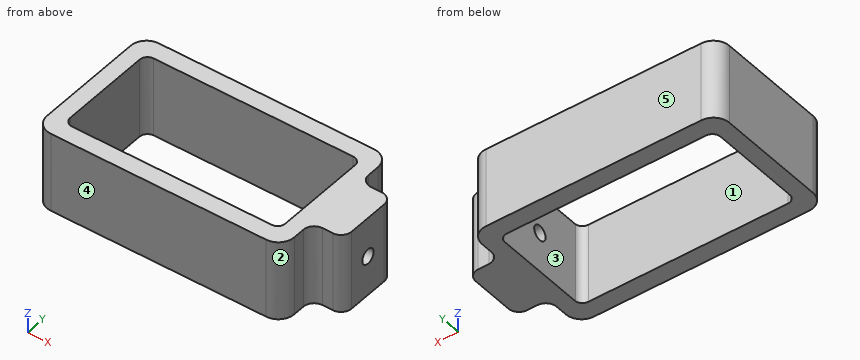
Autodesk Inventor part; units mm, degrees
ref_plane "YZ Plane" through (0, 0, 0) normal (1, 0, 0) x (0, 1, 0)
ref_plane "XZ Plane" through (0, 0, 0) normal (0, 1, 0) x (-1, 0, 0)
ref_plane "Arbeitsebene1" through (0, 0, -15) normal (0, 0, 1) x (1, 0, 0)
sketch "Skizze1" plane through (0, 0, -15) normal (0, 0, 1) x (1, 0, 0)
  line L0 (29.6698, 8.5) -> (29.6698, -8.5)
  arc A0 (29.6698, 8.5) -> (28.1698, 10) centre (28.1698, 8.5) ccw
  line L1 (11.1698, 10) -> (28.1698, 10)
  arc A1 (11.1698, 10) -> (9.6698, 8.5) centre (11.1698, 8.5) ccw
  line L2 (9.6698, -8.5) -> (9.6698, 8.5)
  arc A2 (9.6698, -8.5) -> (11.1698, -10) centre (11.1698, -8.5) ccw
  line L3 (28.1698, -10) -> (11.1698, -10)
  arc A3 (28.1698, -10) -> (29.6698, -8.5) centre (28.1698, -8.5) ccw
  circle A4 centre (27.6698, 8) radius 0.7835
  circle A5 centre (27.6698, -8) radius 0.7835
  circle A6 centre (11.6698, 8) radius 0.7835
  circle A7 centre (11.6698, -8) radius 0.7835
  circle A8 centre (19.6698, 0) radius 7.5
  line L4 (4.2698, 10) -> (4.2698, 8.9)
  line L5 (-5.8302, 10) -> (4.2698, 10)
  line L6 (-5.8302, 8.5) -> (-5.8302, 10)
  arc A9 (-9.3302, 5) -> (-5.8302, 8.5) centre (-9.3302, 8.5) ccw
  line L7 (-10.8302, 5) -> (-9.3302, 5)
  line L8 (-10.8302, -5) -> (-10.8302, 5)
  line L9 (-9.3302, -5) -> (-10.8302, -5)
  arc A10 (-5.8302, -8.5) -> (-9.3302, -5) centre (-9.3302, -8.5) ccw
  line L10 (-5.8302, -10) -> (-5.8302, -8.5)
  line L11 (4.2698, -10) -> (-5.8302, -10)
  line L12 (4.2698, -8.9) -> (4.2698, -10)
  arc A11 (7.6698, -5.5) -> (4.2698, -8.9) centre (7.6698, -8.9) ccw
  line L13 (11.1698, -5.5) -> (7.6698, -5.5)
  line L14 (11.1698, -5) -> (11.1698, -5.5)
  line L15 (11.1698, -5) -> (7.3698, -5)
  line L16 (7.3698, -5) -> (7.3698, 5)
  line L17 (7.3698, 5) -> (11.1698, 5)
  line L18 (11.1698, 5.5) -> (11.1698, 5)
  line L19 (7.6698, 5.5) -> (11.1698, 5.5)
  arc A12 (4.2698, 8.9) -> (7.6698, 5.5) centre (7.6698, 8.9) ccw
  circle A13 centre (-0.8302, 0) radius 2
  line L20 (9.1698, 8.5) -> (9.1698, -8.5)
  arc A14 (9.1698, 8.5) -> (7.6698, 10) centre (7.6698, 8.5) ccw
  line L21 (-9.3302, 10) -> (7.6698, 10)
  arc A15 (-9.3302, 10) -> (-10.8302, 8.5) centre (-9.3302, 8.5) ccw
  line L22 (-10.8302, -8.5) -> (-10.8302, 8.5)
  arc A16 (-10.8302, -8.5) -> (-9.3302, -10) centre (-9.3302, -8.5) ccw
  line L23 (7.6698, -10) -> (-9.3302, -10)
  arc A17 (7.6698, -10) -> (9.1698, -8.5) centre (7.6698, -8.5) ccw
  circle A18 centre (7.1698, 8) radius 0.7835
  circle A19 centre (7.1698, -8) radius 0.7835
  circle A20 centre (-8.8302, 8) radius 0.7835
  circle A21 centre (-8.8302, -8) radius 0.7835
  circle A22 centre (-0.8302, 0) radius 7.5
  line L24 (-9.3302, -5.5) -> (-12.8302, -5.5)
  line L25 (-9.3302, -5) -> (-9.3302, -5.5)
  line L26 (-9.3302, -5) -> (-13.1302, -5)
  line L27 (-13.1302, 5) -> (-9.3302, 5)
  line L28 (-9.3302, 5.5) -> (-9.3302, 5)
  line L29 (-12.8302, 5.5) -> (-9.3302, 5.5)
  line L30 (11.1698, 10) -> (7.6698, 10)
  line L31 (11.1698, -10) -> (7.6698, -10)
  line L32 (-10.858, 10.25) -> (29.642, 10.25)
  line L33 (29.642, 10.25) -> (29.642, -10.25)
  line L34 (29.642, -10.25) -> (-10.858, -10.25)
  line L35 (-10.858, -10.25) -> (-10.858, 10.25)
  line L36 (-10.858, 10.25) -> (29.642, -10.25) construction
  line L37 (29.642, 10.25) -> (-10.858, -10.25) construction
  line L38 (32.642, -10.25) -> (32.642, 10.25)
  line L39 (29.642, 13.25) -> (-10.858, 13.25)
  line L40 (-13.858, 10.25) -> (-13.858, -10.25)
  line L41 (-10.858, -13.25) -> (29.642, -13.25)
  arc A23 (32.642, 10.25) -> (29.642, 13.25) centre (29.642, 10.25) ccw
  arc A24 (29.642, -13.25) -> (32.642, -10.25) centre (29.642, -10.25) ccw
  arc A25 (-13.858, -10.25) -> (-10.858, -13.25) centre (-10.858, -10.25) ccw
  arc A26 (-10.858, 13.25) -> (-13.858, 10.25) centre (-10.858, 10.25) ccw
  line L42 (38.642, 6) -> (32.642, 6)
  line L43 (32.642, 6) -> (32.642, -6)
  line L44 (32.642, -6) -> (38.642, -6)
  line L45 (38.642, -6) -> (38.642, 6)
  line L46 (38.642, 6) -> (32.642, -6) construction
  line L47 (32.642, 6) -> (38.642, -6) construction
  point P0 (0, 0)
  point P1 (9.392, 0)
  point P2 (35.642, 0)
  point P3 (32.642, 0)
  point P4 (29.642, -8.7873)
  point P5 (29.642, 8.7873)
  dimension "d1" = 20.5
  dimension "d2" = 3
  dimension "d3" = 3
  dimension "d6" = 6
  dimension "d7" = 12
extrude "Extrusion1" add sketch "Skizze1" along normal blind 15 contours L0 A3 L33 A0 | A0 L1 L30 L21 L5 A15 L22 L29 L35 L32 L33 | L33 L34 L35 L24 L22 A16 L23 L11 L31 L3 A3 | L29 L22 L27 L35 | L35 L26 L22 L24 | L27 L8 L26 L35 | A24 L41 A25 L40 A26 L39 A23 L38 | L38 L42 L45 L44
fillet "Rundung1" radius 2 4 edges at (32.642, 6, -7.5) (38.642, 6, -7.5) (38.642, -6, -7.5) (32.642, -6, -7.5)
sketch "Skizze2" plane through (38.642, -4, -15) normal (1, 0, 0) x (0, 0, -1)
  line L0 (0, 0) -> (-15, 0)
  line L1 (0, 0) -> (0, 8)
  line L2 (-15, 8) -> (0, 8)
  line L3 (-15, 0) -> (-15, 8)
  circle A0 centre (-7.5, 4) radius 1.4
  point P0 (-15, 4)
  dimension "d9" = 2.8
extrude "Extrusion2" cut sketch "Skizze2" against normal blind 15 contours A0
properties part number "Holisheet_NEMA8_connector"
Source: CAD feature listing. Evaluate the final solid. Frame: model axes, mm. Face numbers are marked on the shaded views. A direction names the side the tool comes from. Give positions to 0.01 mm unless a question says otherwise; leave off trailing zeros. Loops run counter-clockwise (first coordinate to the right, second up) from the corner with the lowest first, then second, coordinate; pieces in that order, holes last. Notation, with made-up numbers: (-25, 12.25) - (23, 12.25) arc R33 cw to (23, 44.25) - close; hole circle Ø9 at (20.25, -35). An arc over 180 degrees is marked (long way). Use CSV: the item, a comma, the result in double quotes. Start each with the question number.
1. Section A-A (x = 26). Output: boundary loops of the cut face in (y, z), then the cut area to 3 significant figures.
2. Ray query, L1, parallel to Y at x = 36, z = -7.5; L2, parallel to Y at x = 27, z = -9.25; L3, parallel to X at y = -3.25, z = -14.25. Return the intervals inside material, ascending.
3. Section B-B (z = -13.5). Output: boundary loops of the cut face in (x, y).
4. Section D-D (z = -7.5). Output: boundary loops of the cut face in (x, y), then the cut area to 3 significant figures.
5. Draft query along Y for the marked faces 3, 4 and 5. Return one class per face: +Y half, -Y half, draft (parallel to the pull), parting line (faces both ways), or undercut.
6. Pin query (flat end, axial travel): pin 1 (2 mm diameter, centred on y = 0, z = -7.5, fed in from +X); pin 2 (1.6 mm diameter, centred on x = 35.5, z = -7.5, fed in from -Y); pin 3 (1.8 mm diameter, centred on y = -8.5, z = -5.5, fed in from +X). Return the tip coordinate at first contact, or that it passes through.
7. Reachability of the marked faces 1 and 2 from +Z, -Z, +X, -X, +Y, -Y: full face, straight path, thin tool, end or side. Return the list, or none.
8. Section C-C (y = 0). Output: boundary loops of the cut face in (x, z).
Response:
1,outline,"(-13.25, -15) - (-10, -15) - (-10, 0) - (-13.25, 0) - close; (10, -15) - (13.25, -15) - (13.25, 0) - (10, 0) - close"
1,area,"97.5 mm²"
2,L1,"-6 to -1.4, 1.4 to 6"
2,L2,"-13.25 to -10, 10 to 13.25"
2,L3,"-13.86 to -10.83, 29.64 to 38.64"
3,outline,"(-13.86, -10.25) arc R3 ccw to (-10.86, -13.25) - (29.64, -13.25) arc R3 ccw to (32.64, -10.25) - (32.64, -8) arc R2 cw to (34.64, -6) - (36.64, -6) arc R2 ccw to (38.64, -4) - (38.64, 4) arc R2 ccw to (36.64, 6) - (34.64, 6) arc R2 cw to (32.64, 8) - (32.64, 10.25) arc R3 ccw to (29.64, 13.25) - (-10.86, 13.25) arc R3 ccw to (-13.86, 10.25) - close; hole (-10.83, -8.5) arc R1.5 ccw to (-9.33, -10) - (28.17, -10) arc R1.5 ccw to (29.64, -8.79) - (29.64, 8.79) arc R1.5 ccw to (28.17, 10) - (-9.33, 10) arc R1.5 ccw to (-10.83, 8.5) - close"
4,outline,"(-13.86, -10.25) arc R3 ccw to (-10.86, -13.25) - (29.64, -13.25) arc R3 ccw to (32.64, -10.25) - (32.64, -8) arc R2 cw to (34.64, -6) - (36.64, -6) arc R2 ccw to (38.64, -4) - (38.64, -1.4) - (29.64, -1.4) - (29.64, -8.79) arc R1.5 cw to (28.17, -10) - (-9.33, -10) arc R1.5 cw to (-10.83, -8.5) - (-10.83, 8.5) arc R1.5 cw to (-9.33, 10) - (28.17, 10) arc R1.5 cw to (29.64, 8.79) - (29.64, 1.4) - (38.64, 1.4) - (38.64, 4) arc R2 ccw to (36.64, 6) - (34.64, 6) arc R2 cw to (32.64, 8) - (32.64, 10.25) arc R3 ccw to (29.64, 13.25) - (-10.86, 13.25) arc R3 ccw to (-13.86, 10.25) - close"
4,area,"464 mm²"
5,face 3,"undercut"
5,face 4,"-Y half"
5,face 5,"+Y half"
6,pin 1,"x = -10.83"
6,pin 2,"y = -6"
6,pin 3,"x = 32.68"
7,face 1,"+Z, -Z"
7,face 2,"+Z, -Z, +X, -Y"
8,outline,"(-13.86, -15) - (-10.83, -15) - (-10.83, 0) - (-13.86, 0) - close; (29.64, -15) - (38.64, -15) - (38.64, -8.9) - (29.64, -8.9) - close; (29.64, -6.1) - (38.64, -6.1) - (38.64, 0) - (29.64, 0) - close"
